from build123d import *

# Parameters (mm, degrees)
ESQUISSE1_R             = 2.6
BOSS_EXTRU_1_DEPTH      = 10
ESQUISSE7_R             = 5.1
ENL_V_MAT_EXTRU_4_DEPTH = 5.4
ESQUISSE4_R             = 2
ENL_V_MAT_EXTRU_2_DEPTH = 10
ENL_V_MAT_EXTRU_3_DEPTH = 11
CONG_1_R                = 5
CONG_2_R                = 4


with BuildPart() as part:
    # Esquisse1 → Boss.-Extru.1 (new body)
    with BuildSketch(Plane(origin=(0, 0, 0), x_dir=(1, 0, 0), z_dir=(0, 1, 0))):
        Polygon((-20, 21), (20, 21), (35, 6), (35, 0), (15, 0), (15, 14), (14, 15), (-14, 15), (-15, 14), (-15, 0), (-35, 0), (-35, 6), align=None)
        with Locations((-22.5, 7.5)):
            Circle(ESQUISSE1_R, mode=Mode.SUBTRACT)
        with Locations((22.5, 7.5)):
            Circle(ESQUISSE1_R, mode=Mode.SUBTRACT)
    extrude(amount=BOSS_EXTRU_1_DEPTH)

    # Esquisse7 → Enlèv. mat.-Extru.4 (cut)
    with BuildSketch(Plane.XZ):
        with Locations((22.5, -7.5)):
            Circle(ESQUISSE7_R)
        with Locations((-22.5, -7.5)):
            Circle(ESQUISSE7_R)
    extrude(amount=-ENL_V_MAT_EXTRU_4_DEPTH, mode=Mode.SUBTRACT)

    # Esquisse4 → Enlèv. mat.-Extru.2 (cut)
    with BuildSketch(Plane.XZ):
        with Locations((19, -16.5)):
            Circle(ESQUISSE4_R)
        with Locations((-19, -16.5)):
            Circle(ESQUISSE4_R)
        with Locations((-31, -4)):
            Circle(ESQUISSE4_R)
        with Locations((31, -4)):
            Circle(ESQUISSE4_R)
    extrude(amount=-ENL_V_MAT_EXTRU_2_DEPTH, mode=Mode.SUBTRACT)

    # Esquisse5 → Enlèv. mat.-Extru.3 (cut, through all)
    with BuildSketch(Plane(origin=(0, 10, 0), x_dir=(1, 0, 0), z_dir=(0, 1, 0))):
        with BuildLine():
            Line((15, 14), (14, 14))
            Line((14, 14), (14, 15))
            ThreePointArc((14, 15), (14.707106781, 14.707106781), (15, 14))
        make_face()
        with BuildLine():
            Line((-14, 14), (-14, 15))
            ThreePointArc((-14, 15), (-14.707106781, 14.707106781), (-15, 14))
            Line((-15, 14), (-14, 14))
        make_face()
    extrude(amount=-ENL_V_MAT_EXTRU_3_DEPTH, mode=Mode.SUBTRACT)

    # Congé1
    cong_1_edges = [part.edges().sort_by_distance(p)[0] for p in [
        (-35, 5, -6),
        (-20, 5, -21),
        (20, 5, -21),
        (35, 5, -6),
    ]]
    fillet(cong_1_edges, radius=CONG_1_R)

    # Congé2
    cong_2_edges = [part.edges().sort_by_distance(p)[0] for p in [
        (35, 5, 0),
        (-35, 5, 0),
    ]]
    fillet(cong_2_edges, radius=CONG_2_R)


solid = part.part
Check sheet for the modelled part. Datum: model origin and axes. Units: mm. A direction names the side the tool comes from. Coordinates: 2 decimals unless noted, no trailing zeros. Loops run counter-clockwise (first coordinate to the right, second up) from the corner with the lowest first, then second, coordinate; pieces in that order, holes last. Notation, with made-up numbers: (17.25, 88) -> (56.25, 88) arc R13 cw to (56.25, 99) -> close; hole circle Ø4 at (41, 79.25). An arc over 180 degrees is marked (long way). Write item = value, one per line. Start each with the question number.
1. Tool access check on faces 1 (the flat face through (15, 5, -7)), 2 (the cylindrical face through (18.74, 4.93, -14.517)), 3 (the flat face through (21, 5.4, -5)). Record the directions out of +Z, -Z, +X, -X, +Y, -Y that give a thin tool (end or side, any length) a straight path to the whole face; none if there is none.
2. Section check C-C on y = 2.25. Give the number of separate pieces and of enclosed holes in the cut face, then the cut area to 3 significant figures.
3. Draft check along Z on faces 4 (the flat face through (0.5, 0, -15.3)), 5 (the flat face through (0, 5, -15)), 6 (the cylindrical face through (18.7, 2.7, -4.1)). Enter one of: released by +Z, released by -Z, zero draft, split by the parting line, or undercut.
4. Section check A-A on x = 22.5. Record the cut outline in (y, z), then the cut area to 3 significant figures.
5. Depth check by flat-ended pin: P1, Ø4.5, axis at x = -22.5, z = -7.5, coming from the +Y side; P2, Ø3, axis at x = -21.5, z = -9, coming from the -Y side; P3, Ø3, axis at y = 7.5, z = -13, coming from the +X side; P4, Ø3, axis at x = -2.5, y = 5, coming from the +Z side. Enter the tip coordinate at first touch or a pass-through.
6. Section check B-B on z = -17.25. Record the cut outline in (x, y).
7. Material ranges on line 1 (X direction, y = 6, z = -16.25); line 2 (X direction, y = 5.5, z = -16); line 3 (Z direction, x = -22.5, y = 7.9), recorded low to high.
8. Section check D-D on x = -19. Record the cut outline in (y, z).
Responses:
q1.face_1 = +Z, +Y, -Y
q1.face_2 = +Y, -Y
q1.face_3 = -Y
q2.separate_pieces = 1
q2.enclosed_holes = 6
q2.area = 573 mm2
q3.face_4 = zero draft
q3.face_5 = released by +Z
q3.face_6 = undercut
q4.outline = (0, -18.5) -> (10, -18.5) -> (10, -10.1) -> (5.4, -10.1) -> (5.4, -12.6) -> (0, -12.6) -> close; (0, -2.4) -> (5.4, -2.4) -> (5.4, -4.9) -> (10, -4.9) -> (10, 0) -> (0, 0) -> close
q4.area = 106 mm2
q5.P1 = through
q5.P2 = 5.4
q5.P3 = 29.5
q5.P4 = -15
q6.outline = (-23.75, 0) -> (-20.85, 0) -> (-20.85, 10) -> (-23.75, 10) -> close; (-17.15, 0) -> (17.15, 0) -> (17.15, 10) -> (-17.15, 10) -> close; (20.85, 0) -> (23.75, 0) -> (23.75, 10) -> (20.85, 10) -> close
q7.line_1 = -24.75 to -20.98, -17.02 to 17.02, 20.98 to 24.75
q7.line_2 = -25 to -20.94, -17.06 to 17.06, 20.94 to 25
q7.line_3 = -18.5 to -10.1, -4.9 to 0
q8.outline = (0, -20.88) -> (10, -20.88) -> (10, -18.5) -> (0, -18.5) -> close; (0, -14.5) -> (10, -14.5) -> (10, 0) -> (0, 0) -> (0, -3.79) -> (5.4, -3.79) -> (5.4, -11.21) -> (0, -11.21) -> close
